Source: CAD feature listing. Evaluate the final solid. Frame: model axes, mm. Face numbers are marked on the shaded views. A direction names the side the tool comes from. Coordinates: 2 decimals unless noted, no trailing zeros. Loops run counter-clockwise (first coordinate to the right, second up) from the corner with the lowest first, then second, coordinate; pieces in that order, holes last. Notation, with made-up numbers: (-24.75, 14) - (34.25, 14) arc R22 cw to (34.25, 47) - close; hole circle Ø10 at (-12, -14). An arc over 180 degrees is marked (long way). Use one line per item in the form item = value. Start each with the question number.
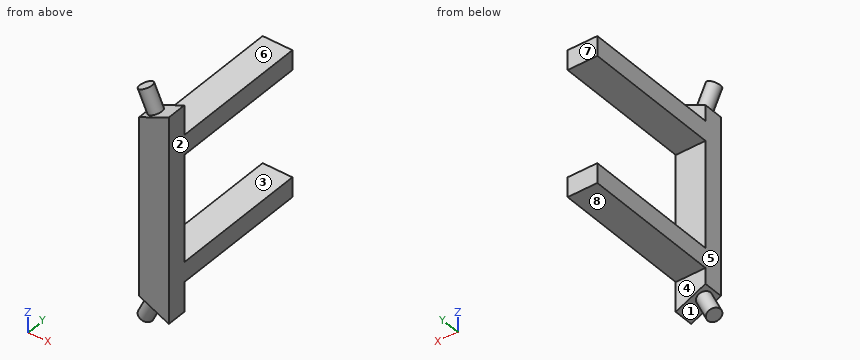
from build123d import *

# Parameters (mm, degrees)
SKETCH1_W           = 38.1
SKETCH1_H           = 25.4
BOSS_EXTRUDE1_DEPTH = 132.08
SKETCH5_W           = 38.1
SKETCH5_H           = 25.4
BOSS_EXTRUDE3_DEPTH = 177.8
CUT_EXTRUDE1_DEPTH  = 25.4
SKETCH3_R           = 8.89
BOSS_EXTRUDE2_DEPTH = 30


with BuildPart() as part:
    # Sketch1 → Boss-Extrude1 (new body)
    with BuildSketch(Plane.XY):
        with Locations((19.05, 12.7)):
            Rectangle(SKETCH1_W, SKETCH1_H)
    boss_extrude1 = extrude(amount=BOSS_EXTRUDE1_DEPTH)

    # Sketch5 → Boss-Extrude3 (add)
    with BuildSketch(Plane(origin=(0, 25.4, 0), x_dir=(1, 0, 0), z_dir=(0, 1, 0))):
        with Locations((19.05, -81.28)):
            Rectangle(SKETCH5_W, SKETCH5_H)
    boss_extrude3 = extrude(amount=BOSS_EXTRUDE3_DEPTH)

    # Sketch2 → Cut-Extrude1 (cut)
    with BuildSketch(Plane(origin=(0, 25.4, 0), x_dir=(1, 0, 0), z_dir=(0, 1, 0))):
        Polygon((-12.106033358, -108.66854216), (38.1, -132.08), (54.824729612, -172.409676007), (-49.386286867, -161.765658866), align=None)
    cut_extrude1 = extrude(amount=-CUT_EXTRUDE1_DEPTH, mode=Mode.SUBTRACT)

    # Mirror2: Boss-Extrude1, Boss-Extrude3, Cut-Extrude1 across plane
    add(boss_extrude1.mirror(Plane(origin=(0, 0, 0), x_dir=(1, 0, 0), z_dir=(0, 0, -1))))
    add(boss_extrude3.mirror(Plane(origin=(0, 0, 0), x_dir=(1, 0, 0), z_dir=(0, 0, -1))))
    add(cut_extrude1.mirror(Plane(origin=(0, 0, 0), x_dir=(1, 0, 0), z_dir=(0, 0, -1))), mode=Mode.SUBTRACT)

    # Sketch3 → Boss-Extrude2 (add)
    with BuildSketch(Plane(origin=(-43.784678988, 0, 93.896547102), x_dir=(0.906307787, 0, 0.422618262), z_dir=(-0.422618262, 0, 0.906307787))):
        with Locations((61.011047984, 12.7)):
            Circle(SKETCH3_R)
    boss_extrude2 = extrude(amount=BOSS_EXTRUDE2_DEPTH)

    # Mirror3: Boss-Extrude2 across plane
    add(boss_extrude2.mirror(Plane.XY))


solid = part.part
(1) Contact query for flat-ended pins moving along their axis: pin 1 (19 mm diameter, centred on x = 14.5, y = 104, fed in from +Z); pin 2 (19 mm diameter, centred on x = 20.5, z = -121.5, fed in from +Y); pin 3 (1 mm diameter, centred on x = 8, y = 150.5, fed in from -Z). Output: stop coordinate, or through.
(2) Access query for the marked faces 1, 2, 3 and 4. Directions: +Z, -Z, +X, -X, +Y, -Y. A direction counts if a zero-diameter tool reaches every point of the face in a straight line with its end or side. Return the directions, or none.
(3) Mould query, pull axis Z, two halves, no side actions, for the marked faces 5, 6, 7 and 8. Classes: +Z half, -Z half, draft (parallel to the pull), parting line (faces both ways), or undercut.
(4) Cut plane D-D, the plane x = 31.5. Output: boundary loops of the cut face in (y, z).
(5) Cut plane B-B, the plane x = 3. State how many separate pieces and enclosed holes the cut face has, plus the area to 3 significant figures.
(6) Cut plane C-C, the plane z = 42.5. Output: boundary loops of the cut face in (x, y).
(7) Material intervals for line 1 (Z direction, x = 32.5, y = 129.5); line 2 (Y direction, x = 23, z = 62); line 3 (Z direction, x = -7, y = 11), sorted ascending.
(8) Cut plane A-A, the plane y = 68.5. Output: boundary loops of the cut face in (x, z).
Recorded:
q1.pin_1 = 93.98
q1.pin_2 = 25.4
q1.pin_3 = -93.98
q2.face_1 = none
q2.face_2 = +Z, -Z, +X, +Y, -Y
q2.face_3 = +X, -X, +Y
q2.face_4 = -Z, +X, -X, +Y
q3.face_5 = undercut
q3.face_6 = +Z half
q3.face_7 = draft
q3.face_8 = -Z half
q4.outline = (0, -129) - (25.4, -129) - (25.4, -93.98) - (203.2, -93.98) - (203.2, -68.58) - (25.4, -68.58) - (25.4, 68.58) - (203.2, 68.58) - (203.2, 93.98) - (25.4, 93.98) - (25.4, 129) - (0, 129) - close
q5.separate_pieces = 3
q5.enclosed_holes = 0
q5.area = 15,900 mm²
q6.outline = (0, 0) - (38.1, 0) - (38.1, 25.4) - (0, 25.4) - close
q7.line_1 = -93.98 to -68.58, 68.58 to 93.98
q7.line_2 = 0 to 25.4
q7.line_3 = -144.15 to -138.73, 138.73 to 144.15
q8.outline = (0, -93.98) - (38.1, -93.98) - (38.1, -68.58) - (0, -68.58) - close; (0, 68.58) - (38.1, 68.58) - (38.1, 93.98) - (0, 93.98) - close
